Here's how the part is built. I have some questions about the finished solid (model axes, mm). Face numbers are marked on the shaded views. A direction names the side the tool comes from. Coordinates: 2 decimals unless noted, no trailing zeros. Order: outer loops, then holes, each group sorted by start corner. A loop starts at its lowest first (then second) coordinate and runs counter-clockwise, first axis right, second up.
```python
from build123d import *

# Parameters (mm, degrees)
F1_DEPTH = 20
F2_R     = 1
F3_R     = 9.99999


# Not quite as in the source:
# - two fillets or chamfers of one size are made in one step
# - a fillet or chamfer is up to 0.001 mm smaller than in the source, because OpenCascade refuses the exact size


with BuildPart() as f1:
    # F0 (on Top) → F1 (new body)
    with BuildSketch(Plane.XY):
        Polygon((-26.4541809829, 58.4762617946), (-26.4541809829, -79.9982637167), (-20.4541809829, -79.9982637167), (-20.4541809829, -54.9982637167), (-12.4541809829, -54.9982637167), (-12.4541809829, -79.9982637167), (-6.4541809829, -79.9982637167), (-6.4541809829, 58.4762617946), (0, 68.5610547662), (0, 90.617305144), (-7.710005641, 90.617305144), (-7.710005641, 70.0017362833), (-27.710005641, 70.0017362833), (-27.710005641, 90.6515493989), (-34.6441827714, 90.6196484681), (-34.6441827714, 68.5610547662), align=None)
    extrude(amount=F1_DEPTH)

    # F2
    f2_edges = [f1.edges().sort_by_distance(p)[0] for p in [
        (-26.454181, -79.998264, 10),
        (-6.454181, -79.998264, 10),
        (-27.710006, 90.651549, 10),
        (-34.644183, 90.619648, 10),
        (-26.454181, 58.476262, 10),
        (-6.454181, 58.476262, 10),
        (0, 90.617305, 10),
        (-7.710006, 90.617305, 10),
    ]]
    fillet(f2_edges, radius=F2_R)

    # F3 (radius 10 in the source; OpenCascade refuses exactly that, so slightly less here)
    f3_edges = [f1.edges().sort_by_distance(p)[0] for p in [
        (-7.710006, 70.001736, 10),
        (-27.710006, 70.001736, 10),
    ]]
    fillet(f3_edges, radius=F3_R)


solid = f1.part
```
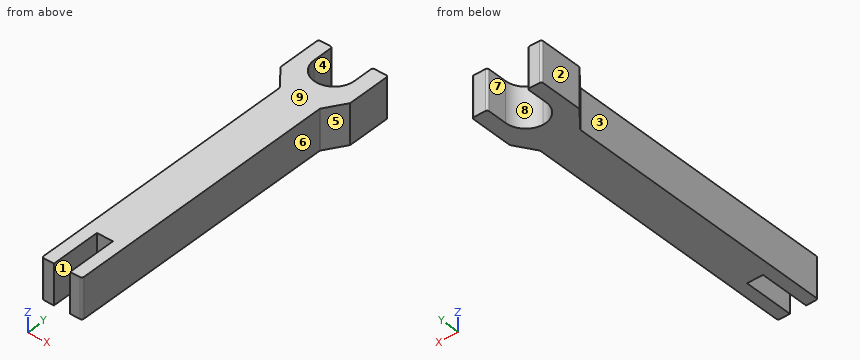
Q1. Will these pins go through, and if not, where does the flat tip stop? pin 1 (5 mm diameter, centred on x = -18.5, z = 6, fed in from +Y); pin 2 (3 mm diameter, centred on x = -4.5, z = 9, fed in from +Y); pin 3 (4 mm diameter, centred on x = -29, y = 1.5, fed in from +Z); pin 4 (2 mm diameter, centred on x = -20.5, z = 12, fed in from +Y).
Q2. We'd pull the mould along X, two halves only. Please class the marked faces 6, 7, 8 and 9: pulls with the +X half, pulls with the -X half, needs draft (parallel to the pull), parting line crosses it, or undercut.
Q3. I need wall thicknesses on L1, parallel to X at y = 80.5, z = 13; L2, parallel to X at y = -2.5, z = 14.75; L3, parallel to X at y = -64.5, z = 5.25. Which ranges of each line are inside material? Lowest first, please.
Q4. If we section it at C-C on y = -26: Write out the boundary of the cut face in (x, z), then the cut area to 3 significant figures.
Q5. If we section it at B-B on y = 74.5: Write out the boundary of the cut face in (x, z).
Q6. For the marked faces 1, 2, 3, 4 and 5, which set-ups out of +Z, -Z, +X, -X, +Y, -Y let a thin tool reach every point of the face, with its end or its side?
Reply:
1. pin 1: stops at y = 70.56
1. pin 2: stops at y = 90.62
1. pin 3: passes through
1. pin 4: stops at y = 70.75
2. face 6: pulls with the +X half
2. face 7: undercut
2. face 8: undercut
2. face 9: needs draft
3. L1: x = -34.64 to -27.71, -7.71 to 0
3. L2: x = -26.45 to -6.45
3. L3: x = -26.45 to -20.45, -12.45 to -6.45
4. outline: (-26.45, 0) - (-6.45, 0) - (-6.45, 20) - (-26.45, 20) - close
4. area: 400 mm2
5. outline: (-34.64, 0) - (-26.06, 0) - (-26.06, 20) - (-34.64, 20) - close; (-9.36, 0) - (0, 0) - (0, 20) - (-9.36, 20) - close
6. face 1: +Z, -Z, -Y
6. face 2: +Z, -Z, -X, +Y, -Y
6. face 3: +Z, -Z, -X, -Y
6. face 4: +Z, -Z, +Y
6. face 5: +Z, -Z, +X, -Y
